from build123d import *

# Parameters (mm, degrees)
F1_DEPTH = 279.4
F3_DEPTH = 76.2


with BuildPart() as f1:
    # F0 (on Right) → F1 (new body)
    with BuildSketch(Plane.YZ):
        with BuildLine():
            Line((-101.6, -114.072286), (-101.6, -215.672286))
            Line((-101.6, -215.672286), (-12.7, -215.672286))
            Line((-12.7, -215.672286), (-12.7, -288.716509))
            Line((-12.7, -288.716509), (63.5, -288.716509))
            Line((63.5, -288.716509), (63.5, -215.672286))
            Line((63.5, -215.672286), (50.8, -215.672286))
            Line((50.8, -215.672286), (50.8, -276.016509))
            Line((50.8, -276.016509), (0, -276.016509))
            Line((0, -276.016509), (0, -215.672286))
            ThreePointArc((0, -215.672286), (-29.757951, -143.830237), (-101.6, -114.072286))
        make_face()
    extrude(amount=F1_DEPTH)

    # F2 (on face) → F3 (join)
    with BuildSketch(Plane(origin=(0, 63.5, 0), x_dir=(-1, 0, 0), z_dir=(0, 1, 0))):
        with BuildLine():
            ThreePointArc((279.4, -276.016509), (139.7, -415.716509), (0, -276.016509))
            Line((0, -276.016509), (-6.35, -276.016509))
            ThreePointArc((-6.35, -276.016509), (139.7, -422.066509), (285.75, -276.016509))
            Line((285.75, -276.016509), (279.4, -276.016509))
        make_face()
    extrude(amount=-F3_DEPTH)


solid = f1.part
Part model, mm, in its own coordinate system. A direction names the side the tool comes from. Coordinates: 2 decimals unless noted, no trailing zeros. Order: outer loops, then holes, each group sorted by start corner. A loop starts at its lowest first (then second) coordinate and runs counter-clockwise, first axis right, second up. Notation, with made-up numbers: M -40,-4.5 L -9,-4.5 A24 cw -9,24.5 Z; hole C 10,-13.5 d1. An arc over 180 degrees is marked long. One line per question, with ' | ' between items.
Q1. Slice it at B-B (z = -133). Give the cut face in (x, y).
A:
outline: M 0,-101.6 L 279.4,-101.6 L 279.4,-42.54 L 0,-42.54 Z
Q2. Two-plate mould, pull along X, no slides. Class faces 1 (the face through (138, 50.8, -245)), 2 (the face through (-142.93, 25.93, -422.03)), 3 (the face through (-142.772, 25.933, -415.683)): +X half, -X half, draft (parallel to the pull), parting line (faces both ways), or undercut.
A:
face 1: draft | face 2: parting line | face 3: undercut
Q3. Pin check, flat tips, straight feed: P1, Ø4, axis at y = 58, z = -260.5, coming from the -X side; P2, Ø12, axis at y = 40.5, z = -301.5, coming from the -X side; P3, Ø5, axis at x = -282.5, y = 19.5, coming from the +Z side; P4, Ø10, axis at y = -19, z = -365.5, coming from the +X side. Stop position of each tip, or through.
A:
P1: stops at x = 0 | P2: stops at x = -284.44 | P3: stops at z = -276.02 | P4: passes through
Q4. Slice it at C-C (x = -139.7). Give the cut face in (y, z).
A:
outline: M -12.7,-422.07 L 63.5,-422.07 L 63.5,-415.72 L -12.7,-415.72 Z
Q5. Drill centre lines: line 1 (Y direction, x = 67.5, z = -252); line 2 (X direction, y = -9, z = -256); line 3 (Z direction, x = 171, y = 29.5). Where is each one in solid material? Low to high.
A:
line 1: y = -12.7 to 0, 50.8 to 63.5 | line 2: x = 0 to 279.4 | line 3: z = -288.72 to -276.02
Q6. 3-axis set-ups, long thin cutter, end or side, ignore diameter. For faces 4 (the face through (141, 25, -288.717)), 5 (the face through (0, 57, -245)), 6 (the face through (138, 26, -276.017)), 7 (the face through (124, -12.7, -265)): which of +Z, -Z, +X, -X, +Y, -Y reach the whole face in a straight line?
A:
face 4: -Z, +X, +Y, -Y | face 5: +Z, -X, +Y, -Y | face 6: +Z, +X, -X | face 7: -Z, +X, -X, -Y
Q7. Slice it at A-A (x = 105). Give the cut face in (y, z), and give its area (3 significant figures).
A:
outline: M -101.6,-215.67 L -12.7,-215.67 L -12.7,-288.72 L 63.5,-288.72 L 63.5,-215.67 L 50.8,-215.67 L 50.8,-276.02 L 0,-276.02 L 0,-215.67 A101.6 ccw -101.6,-114.07 Z | area: 10,600 mm^2
